Source: CAD feature listing. Evaluate the final solid. Frame: model axes, mm. Face numbers are marked on the shaded views. Coordinates: 2 decimals unless noted, no trailing zeros. Write each loop counter-clockwise with the first axis right and the second up, starting at its lowest first coordinate (ties: lowest second). Pieces come first, ordered by that corner, then holes. Notation, with made-up numbers: M 55,-10 L 98,-10 A20 cw 98,-4 Z; hole C 8.5,84.5 d10. An arc over 180 degrees is marked long. One line per item, written item: value. Start each with the question number.
Item 1: Cut plane B-B, the plane x = -14.5. Output: boundary loops of the cut face in (y, z), then the cut area to 3 significant figures.
Item 2: Pin query (flat end, axial travel): P1, Ø2, axis at x = 13, z = 26, coming from the -Y side. Return the tip coordinate at first contact, or that it passes through.
Item 3: Cut plane D-D, the plane y = -3.25. Output: boundary loops of the cut face in (x, z), then the cut area to 3 significant figures.
Item 4: Cut plane A-A, the plane z = 0. Output: boundary loops of the cut face in (x, y), then the cut area to 3 significant figures.
Item 5: Ray query, L1, parallel to X at y = -2, z = 0; L2, parallel to X at y = -4.65, z = 22.5; L3, parallel to Z at x = -16.5, y = -1.3. Return the intervals inside material, ascending. Write a range as from..to.
Item 6: Mould query, pull axis X, two halves, no side actions, for the marked faces 1, 2 and 3. Classes: released by +X, released by -X, zero draft, split by the parting line, or undercut.
Item 7: Cut plane C-C, the plane x = -29. Output: boundary loops of the cut face in (y, z), then the cut area to 3 significant figures.
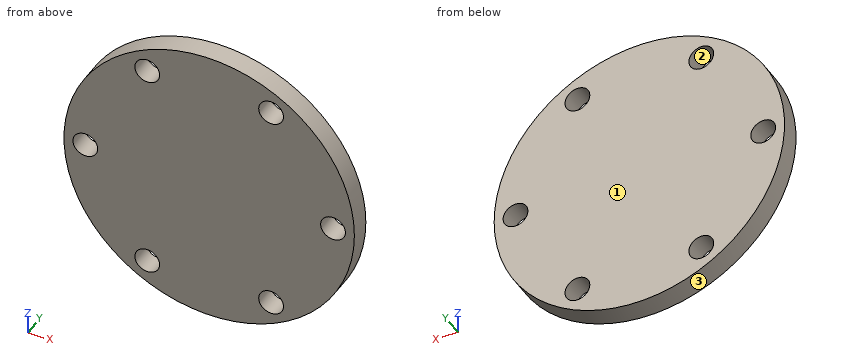
Autodesk Fusion 360 part; units mm, degrees
sketch "Sketch1" plane through (0, 0, 0) normal (0, 1, 0) x (1, 0, 0)
  circle A0 centre (0, 0) radius 34
  circle A1 centre (0, 0) radius 29 construction
  point P0 (-29, 0)
  dimension "d1" = 68
  dimension "d2" = 58
extrude "Extrude1" add sketch "Sketch1" against normal blind 5
hole "Hole1" at (-29, 0, 0) direction (0, -1, 0) diameter 5.8 end through all
pattern_circular "C-Pattern1" count 6 over 360 about axis through (0, 1.75, 0) along (0, 1, 0) of "Hole1"
From the geometry:
1. outline: M -5,-30.75 L 0,-30.75 L 0,-28.01 L -5,-28.01 Z; M -5,-22.21 L 0,-22.21 L 0,22.21 L -5,22.21 Z; M -5,28.01 L 0,28.01 L 0,30.75 L -5,30.75 Z
1. area: 250 mm²
2. P1: passes through
3. outline: C 0,0 d68; hole C -29,0 d5.8; hole C -14.5,-25.11 d5.8; hole C -14.5,25.11 d5.8; hole C 14.5,-25.11 d5.8; hole C 14.5,25.11 d5.8; hole C 29,0 d5.8
3. area: 3,470 mm²
4. outline: M -34,-5 L -31.9,-5 L -31.9,0 L -34,0 Z; M -26.1,-5 L 26.1,-5 L 26.1,0 L -26.1,0 Z; M 31.9,-5 L 34,-5 L 34,0 L 31.9,0 Z
4. area: 282 mm²
5. L1: x = -34..-31.9, -26.1..26.1, 31.9..34
5. L2: x = -25.49..-15.75, -13.25..13.25, 15.75..25.49
5. L3: z = -29.73..-27.21, -23.01..23.01, 27.21..29.73
6. face 1: zero draft
6. face 2: undercut
6. face 3: split by the parting line
7. outline: M -5,-17.75 L 0,-17.75 L 0,-2.9 L -5,-2.9 Z; M -5,2.9 L 0,2.9 L 0,17.75 L -5,17.75 Z
7. area: 148 mm²
